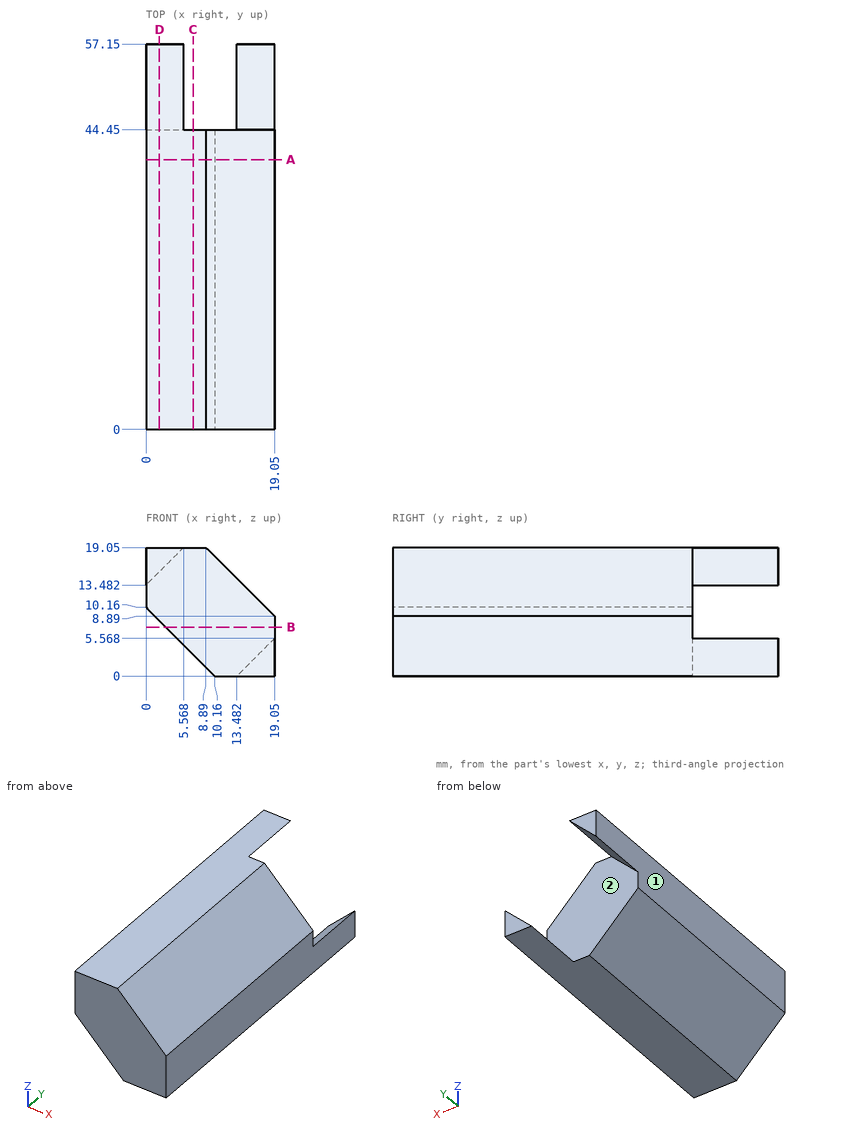
Here's the drawing with two shaded views (mm, measured from the low corner). I have some questions. A direction names the side the tool comes from. Coordinates: 2 decimals unless noted, no trailing zeros. Write each loop counter-clockwise with the first axis right and the second up, starting at its lowest first coordinate (ties: lowest second). Pieces come first, ordered by that corner, then holes. Notation, with made-up numbers: M 13,13.5 L 31,13.5 A17 cw 31,39.5 Z; hole C 77,64 d2. An arc over 180 degrees is marked long. Write item = value, one per line. Start each with the question number.
Q1. If we section it at C-C, the plane x = 7: Write out the boundary of the cut face in (y, z).
Q2. On a 3-axis mill with a long thin cutter (end or side, diameter ignored), from which of +Z, -Z, +X, -X, +Y, -Y can I reach the whole of each face in a straight line? I mean the marked faces 1 and 2. Say none if no direction works.
Q3. If we section it at D-D, the plane x = 2: Write out the boundary of the cut face in (y, z).
Q4. If we section it at A-A, the plane y = 40: Write out the boundary of the cut face in (x, z), then the cut area to 3 significant figures.
Q5. If I drill on L1, parallel to Y at x = 6.75, z = 16; L2, parallel to Z at x = 18, y = 11; L3, parallel to Z at x = 6.75, y = 38, over which ranges is the centre line in solid material (lowest first)? Write a range as [from, to].
Q6. If we section it at B-B, the plane z = 7.25: Write out the boundary of the cut face in (x, y).
Q7. I'm going to push a flat-ended pin straight in: pin 1 (10 mm diameter, centred on x = 16.5, z = 13.5, fed in from +Y). Where does the tip first touch, or does it pass through?
Check sheet entries:
q1.outline = M 0,3.16 L 44.45,3.16 L 44.45,19.05 L 0,19.05 Z
q2.face_1 = +Z, -Z, -X, +Y, -Y
q2.face_2 = +Y
q3.outline = M 0,8.16 L 44.45,8.16 L 44.45,15.48 L 57.15,15.48 L 57.15,19.05 L 0,19.05 Z
q4.outline = M 0,10.16 L 10.16,0 L 19.05,0 L 19.05,8.89 L 8.89,19.05 L 0,19.05 Z
q4.area = 260 mm²
q5.L1 = [0, 44.45]
q5.L2 = [0, 9.94]
q5.L3 = [3.41, 19.05]
q6.outline = M 2.91,0 L 19.05,0 L 19.05,44.45 L 2.91,44.45 Z
q7.pin_1 = 44.45
